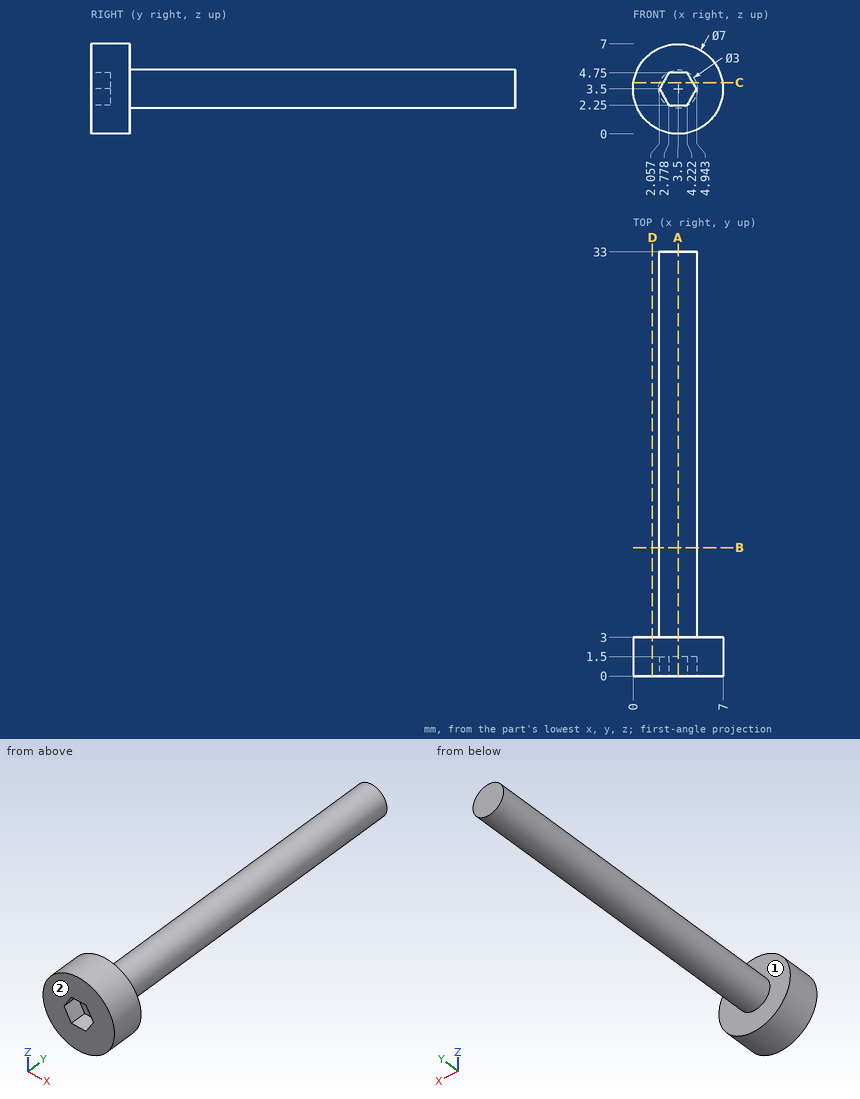
Can you work these out from the drawing? Everything is in mm from the part's minimum corner. A direction names the side the tool comes from. Give positions to 0.01 mm unless a question says otherwise; leave off trailing zeros. Order: outer loops, then holes, each group sorted by start corner. A loop starts at its lowest first (then second) coordinate and runs counter-clockwise, first axis right, second up.
1. For the marked faces 1 and 2, which set-ups out of +Z, -Z, +X, -X, +Y, -Y let a thin tool reach every point of the face, with its end or its side?
2. Will these pins go through, and if not, where does the flat tip stop? P1, Ø3, axis at x = 2.5, y = 10, coming from the +Z side; P2, Ø1.5, axis at y = 22.5, z = 3.5, coming from the +X side; P3, Ø1.5, axis at x = 1.5, z = 4.5, coming from the -Y side.
3. I need wall thicknesses on L1, parallel to Y at x = 3, z = 3; L2, parallel to Y at x = 5.25, z = 5.75; L3, parallel to X at y = 31, z = 3.5. Which ranges of each line are inside material? Lowest first, please.
4. Suppose I cut it at A-A (x = 3.5). List the corners of the cut face in (y, z) for me.
5. Suppose I cut it at B-B (y = 10). List the corners of the cut face in (x, z) for me.
6. Suppose I cut it at D-D (x = 1.5). List the corners of the cut face in (y, z) for me.
7. Suppose I cut it at C-C (z = 4). List the corners of the cut face in (x, y) for me (1 decimal).
Solved:
1. face 1: +Y
1. face 2: +Z, -Z, +X, -X, -Y
2. P1: stops at z = 5
2. P2: stops at x = 5
2. P3: stops at y = 0
3. L1: y = 1.5 to 33
3. L2: y = 0 to 3
3. L3: x = 2 to 5
4. outline: (0, 0) - (3, 0) - (3, 2) - (33, 2) - (33, 5) - (3, 5) - (3, 7) - (0, 7) - (0, 4.75) - (1.5, 4.75) - (1.5, 2.25) - (0, 2.25) - close
5. outline: circle Ø3 at (3.5, 3.5)
6. outline: (0, 0.63) - (3, 0.63) - (3, 6.37) - (0, 6.37) - close
7. outline: (0, 0) - (2.3, 0) - (2.3, 1.5) - (4.7, 1.5) - (4.7, 0) - (7, 0) - (7, 3) - (4.9, 3) - (4.9, 33) - (2.1, 33) - (2.1, 3) - (0, 3) - close
